Geometry: final body of the model. Coordinates: model frame, mm. A direction names the side the tool comes from. Give positions to 0.01 mm unless a question says otherwise; leave off trailing zeros. Loops run counter-clockwise (first coordinate to the right, second up) from the corner with the lowest first, then second, coordinate; pieces in that order, holes last. Notation, with made-up numbers: (0.5, 72.5) -> (6.5, 72.5) arc R31 ccw to (6.5, 107.5) -> close; hole circle Ø9 at (0, 0). An arc over 180 degrees is marked (long way). One line per item, written item: value. Start each with the question number.
from build123d import *
from build123d.topology import SkipClean

# Parameters (mm, degrees)
SKETCH1_R           = 205
BOSS_EXTRUDE1_DEPTH = 705
CUT_EXTRUDE14_DEPTH = 210
SHELL1_T            = -5
CUT_EXTRUDE15_DEPTH = 170
CUT_EXTRUDE16_DEPTH = 60
SKETCH22_R          = 202.5
SKETCH22_R_2        = 200
BOSS_EXTRUDE4_DEPTH = 20
SKETCH26_R          = 3
CUT_EXTRUDE18_DEPTH = 781.81687994
CIRPATTERN1_COUNT   = 4
CIRPATTERN1_ANGLE   = 135


with BuildPart() as part:
    # Sketch1 → Boss-Extrude1 (new body)
    with BuildSketch(Plane(origin=(0, 0, 0), x_dir=(1, 0, 0), z_dir=(0, 1, 0))):
        with Locations(Location((0, 0, 0), (0, 0, 270))):
            Circle(SKETCH1_R)
    extrude(amount=BOSS_EXTRUDE1_DEPTH)

    # Sketch17 → Cut-Extrude14 (cut)
    with BuildSketch(Plane(origin=(0, 0, 0), x_dir=(1, 0, 0), z_dir=(0, 1, 0))):
        with BuildLine():
            Line((-204.022057631, -20), (204.022057631, -20))
            ThreePointArc((204.022057631, -20), (0, -205), (-204.022057631, -20))
        make_face()
    extrude(amount=CUT_EXTRUDE14_DEPTH, mode=Mode.SUBTRACT)

    # Shell1
    shell1_openings = [part.faces().sort_by_distance(p)[0] for p in [
        (0, 705, 0),
        (0, 105, 20),
        (0, 210, 97.908161043),
        (0, 0, -76.302369803),
    ]]
    offset(amount=SHELL1_T, openings=shell1_openings)

    # Sketch18 → Cut-Extrude15 (cut)
    with BuildSketch(Plane(origin=(0, 675, 0), x_dir=(1, 0, 0), z_dir=(0, 1, 0))):
        with BuildLine():
            Line((-205, 0), (205, 0))
            ThreePointArc((205, 0), (0, -205), (-205, 0))
        make_face()
    extrude(amount=-CUT_EXTRUDE15_DEPTH, mode=Mode.SUBTRACT)

    # Sketch19 → Cut-Extrude16 (cut)
    with BuildSketch(Plane(origin=(0, 260, 0), x_dir=(-1, 0, 0), z_dir=(0, -1, 0))):
        with BuildLine():
            Line((-205, 0), (205, 0))
            ThreePointArc((205, 0), (0, 205), (-205, 0))
        make_face()
    extrude(amount=CUT_EXTRUDE16_DEPTH, mode=Mode.SUBTRACT)

    # Sketch22 → Boss-Extrude4 (add)
    with BuildSketch(Plane(origin=(0, 705, 0), x_dir=(1, 0, 0), z_dir=(0, 1, 0))):
        with Locations(Location((0, 0, 0), (0, 0, 270))):
            Circle(SKETCH22_R)
        with Locations(Location((0, 0, 0), (0, 0, 354.260829523))):
            Circle(SKETCH22_R_2, mode=Mode.SUBTRACT)
    extrude(amount=BOSS_EXTRUDE4_DEPTH)

    # Sketch26 → Cut-Extrude18 (cut, symmetric)
    with SkipClean():  # the faces are left unmerged after this step: merging them gives an invalid solid
        with BuildSketch(Plane.XY):
            with Locations((0, 715)):
                Circle(SKETCH26_R)
        cut_extrude18 = extrude(amount=CUT_EXTRUDE18_DEPTH, both=True, mode=Mode.SUBTRACT)

    # CirPattern1: Cut-Extrude18 ×4 about axis
    with SkipClean():  # the faces are left unmerged after this step: merging them gives an invalid solid
        cirpattern1_axis = Axis((0, 832.537864543, 0), (0, -1, 0))
        for i in range(1, CIRPATTERN1_COUNT):
            add(cut_extrude18.rotate(cirpattern1_axis, i * CIRPATTERN1_ANGLE / (CIRPATTERN1_COUNT - 1)), mode=Mode.SUBTRACT)


solid = part.part
Item 1: Ray query, line 1 along Y through (x, z) = (0, -201.25); line 2 along X through (y, z) = (384, 0); line 3 along Z through (x, y) = (184, 481). Return the intervals inside material, ascending. Write a range as [from, to].
Item 2: Section B-B, the plane z = -104. Output: boundary loops of the cut face in (x, y).
Item 3: Mould query, pull axis Z, two halves, no side actions, for faces 1 (the face through (-197.685, 714.86, -43.898)), 2 (the face through (35.9, 357.42, -196.75)), 3 (the face through (16, 505, 201)). Classes: pulls with the +Z half, pulls with the -Z half, needs draft (parallel to the pull), parting line crosses it, or undercut.
Item 4: Pin query (flat end, axial travel): pin 1 (8 mm diameter, centred on x = -60.5, y = 536.5, fed in from +Z); pin 2 (1 mm diameter, centred on x = -149.5, y = 128, fed in from +Z); pin 3 (9.5 mm diameter, centred on y = 715, z = 0, fed in from +X); pin 4 (3.5 mm diameter, centred on y = 715, z = 0, fed in from +X). Return the tip coordinate at first contact, or that it passes through.
Item 5: Access query for faces 4 (the face through (1, 260, -202)), 5 (the face through (16, 675, 201)), 6 (the face through (47, 705, -198)). Directions: +Z, -Z, +X, -X, +Y, -Y. A direction counts if a zero-diameter tool reaches every point of the face in a straight line with its end or side. Return the directions, or none.
Item 6: Section C-C, the plane y = 390.5. Output: boundary loops of the cut face in (x, z), then the cut area to 3 significant figures.
Item 7: Section D-D, the plane x = -68. Output: boundary loops of the cut face in (y, z).
Geometry check:
1. line 1: y = [0, 200], [260, 712], [718, 725]
1. line 2: x = [-205, -200], [200, 205]
1. line 3: z = [-90.38, -78.38], [78.38, 90.38]
2. outline: (-176.66, 0) -> (-170.83, 0) -> (-170.83, 200) -> (-176.66, 200) -> close; (-176.66, 260) -> (-170.83, 260) -> (-170.83, 725) -> (-173.75, 725) -> (-173.75, 705) -> (-176.66, 705) -> close; (170.83, 0) -> (176.66, 0) -> (176.66, 200) -> (170.83, 200) -> close; (170.83, 260) -> (176.66, 260) -> (176.66, 705) -> (173.75, 705) -> (173.75, 725) -> (170.83, 725) -> close
3. face 1: parting line crosses it
3. face 2: undercut
3. face 3: needs draft
4. pin 1: stops at z = -189.31
4. pin 2: stops at z = -132.29
4. pin 3: stops at x = 202.5
4. pin 4: passes through
5. face 4: -Z, +X, -X
5. face 5: +Z, +X, -X
5. face 6: +Y
6. outline: circle Ø410 at (0, 0); hole circle Ø400 at (0, 0)
6. area: 6,360 mm2
7. outline: (0, -193.39) -> (200, -193.39) -> (200, -188.09) -> (0, -188.09) -> close; (210, 188.09) -> (505, 188.09) -> (505, 193.39) -> (210, 193.39) -> close; (260, -193.39) -> (705, -193.39) -> (705, -190.74) -> (725, -190.74) -> (725, -188.09) -> (260, -188.09) -> close; (675, 188.09) -> (725, 188.09) -> (725, 190.74) -> (705, 190.74) -> (705, 193.39) -> (675, 193.39) -> close
